Geometry: final body of the model. Coordinates: model frame, mm. Face numbers are marked on the shaded views. Give positions to 0.01 mm unless a question says otherwise; leave off trailing zeros. Order: outer loops, then holes, each group sorted by start corner. A loop starts at its lowest first (then second) coordinate and runs counter-clockwise, first axis right, second up. Notation, with made-up numbers: (25, -25.5) -> (29, -25.5) arc R26 ccw to (29, 13.5) -> close; hole circle Ø3 at (-3, 70.25). An arc over 180 degrees is marked (long way). One line per question, with ' | ' between items. Start each with the question number.
(1) First-contact query: pin 1 Ø3 at (y, z) = (24.15, 4.76) entering from +X; pin 2 Ø3.5 at (y, z) = (1.92, 4.76) entering from -X; pin 3 Ø1.5 at (y, z) = (24, 4) entering from -X. Flat tips, straight axial feed; report the tip coordinate or a pass-through.
(2) Mould query, pull axis X, two halves, no side actions, for the marked faces 1, 2 and 3. Classes: +X half, -X half, draft (parallel to the pull), parting line (faces both ways), or undercut.
(3) Section D-D (x = -211.5). Return loops of the section in (y, z) (1 decimal).
(4) Section B-B (y = 13.5). Return loops of the section in (x, z) (1 decimal), then the cut area to 3 significant figures.
(5) Section C-C (x = -220.5). Return loops of the section in (y, z) (1 decimal).
(6) Ray query, L1, parallel to Y at x = -223, z = 4.25; L2, parallel to Y at x = -245, z = 5.5; L3, parallel to X at y = 45, z = 3. Return the intervals inside material, ascending.
(7) Section A-A (z = 1.5). Return loops of the section in (x, y) (1 decimal).
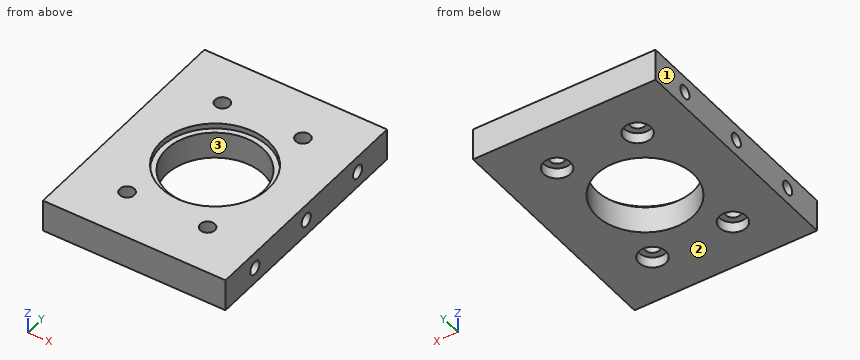
Autodesk Inventor part; units mm, degrees
ref_plane "Work Plane1" through (-222.5199, -10.7756, 0) normal (1, 0, 0) x (0, 0, -1)
ref_plane "YZ Plane" through (0, 0, 0) normal (1, 0, 0) x (0, 1, 0)
ref_plane "XZ Plane" through (0, 0, 0) normal (0, 1, 0) x (-1, 0, 0)
sketch "Sketch1" plane through (0, 0, 0) normal (0, 0, 1) x (1, 0, 0)
  circle A0 centre (0, 0) radius 38.1 construction
  circle A1 centre (0, 0) radius 41.275 construction
  line L0 (-7.3323, 0) -> (-3.6662, 6.35) construction
  line L1 (-3.6662, 6.35) -> (3.6662, 6.35) construction
  line L2 (3.6662, 6.35) -> (7.3323, 0) construction
  line L3 (7.3323, 0) -> (3.6662, -6.35) construction
  line L4 (3.6662, -6.35) -> (-3.6662, -6.35) construction
  line L5 (-3.6662, -6.35) -> (-7.3323, 0) construction
  circle A2 centre (0, 0) radius 14.2875 construction
  circle A3 centre (0, 0) radius 15.875 construction
  circle A4 centre (0, 0) radius 8.7313 construction
  circle A5 centre (0, 0) radius 22.225 construction
  line L6 (34.925, 38.1) -> (34.925, 95.25) construction
  line L7 (34.925, 95.25) -> (-34.925, 95.25) construction
  line L8 (-34.925, 95.25) -> (-34.925, 38.1) construction
  line L9 (34.925, 38.1) -> (-34.925, 38.1) construction
  line L10 (34.925, 38.1) -> (21.2491, -6.5137) construction
  line L11 (-34.925, 38.1) -> (-21.2491, -6.5137) construction
  circle A6 centre (-30.353, 38.1) radius 3.9624 construction
  line L12 (53.34, 95.25) -> (-53.34, 95.25) construction
  line L13 (-53.34, 95.25) -> (-53.34, 104.775) construction
  line L14 (-53.34, 104.775) -> (53.34, 104.775) construction
  line L15 (53.34, 104.775) -> (53.34, 95.25) construction
  circle A7 centre (-222.5199, 24.1494) radius 53.34 construction
  line L16 (-190.7699, 59.0744) -> (-254.2699, 59.0744)
  line L17 (-254.2699, 59.0744) -> (-254.2699, -10.7756)
  line L18 (-254.2699, -10.7756) -> (-190.7699, -10.7756)
  line L19 (-190.7699, -10.7756) -> (-190.7699, 59.0744)
  line L20 (-195.5324, 59.0744) -> (-195.5324, -10.7756)
  line L21 (-249.5074, 59.0744) -> (-249.5074, -10.7756)
  line L22 (-209.8199, 68.5994) -> (-235.2199, 68.5994) construction
  line L23 (-235.2199, 68.5994) -> (-235.2199, -20.3006) construction
  line L24 (-235.2199, -20.3006) -> (-209.8199, -20.3006) construction
  line L25 (-209.8199, -20.3006) -> (-209.8199, 68.5994) construction
  line L26 (34.925, 88.9) -> (-34.925, 88.9) construction
  circle A8 centre (30.353, 38.1) radius 3.9624 construction
  circle A9 centre (30.353, 76.2) radius 3.9624 construction
  circle A10 centre (-30.353, 76.2) radius 3.9624 construction
  circle A11 centre (0, 47.625) radius 3.9624 construction
  line L27 (34.925, 92.075) -> (-34.925, 92.075) construction
  circle A12 centre (0, 71.755) radius 14.2875 construction
  circle A13 centre (0, 71.755) radius 15.875 construction
  line L28 (7.3323, 71.755) -> (3.6662, 65.405) construction
  line L29 (3.6662, 65.405) -> (-3.6662, 65.405) construction
  line L30 (-3.6662, 65.405) -> (-7.3323, 71.755) construction
  line L31 (-7.3323, 71.755) -> (-3.6662, 78.105) construction
  line L32 (-3.6662, 78.105) -> (3.6662, 78.105) construction
  line L33 (3.6662, 78.105) -> (7.3323, 71.755) construction
  point P0 (22.225, 92.075)
  point P1 (0, 92.075)
  point P2 (-22.225, 92.075)
  point P3 (0, 47.625)
  dimension "d0" = 76.2
  dimension "d2" = 82.55
  dimension "d3" = 12.7
  dimension "d4" = 28.575
  dimension "d5" = 31.75
  dimension "d6" = 17.4625
  dimension "d7" = 44.45
  dimension "d8" = 69.85
  dimension "d9" = 34.925
  dimension "d10" = 38.1
  dimension "d11" = 57.15
  dimension "d13" = 7.9248
  dimension "d14" = 9.525
  dimension "d15" = 106.68
  dimension "d16" = 53.34
  dimension "d17" = 106.68
  dimension "d18" = 69.85
  dimension "d19" = 34.925
  dimension "d20" = 63.5
  dimension "d21" = 31.75
  dimension "d22" = 4.7625
  dimension "d23" = 4.7625
  dimension "d24" = 25.4
  dimension "d25" = 14.2875
  dimension "d26" = 88.9
  dimension "d27" = 14.2875
  dimension "d28" = 44.45
  dimension "d29" = 4.572
  dimension "d30" = 6.35
  dimension "d31" = 0
  dimension "d32" = 7.9248
  dimension "d33" = 4.572
  dimension "d34" = 7.9248
  dimension "d35" = 7.9248
  dimension "d36" = 4.572
  dimension "d37" = 4.572
  dimension "d38" = 38.1
  dimension "d39" = 38.1
  dimension "d40" = 7.9248
  dimension "d41" = 9.525
  dimension "d42" = 34.925
  dimension "d44" = 3.175
  dimension "d45" = 34.925
  dimension "d46" = 12.7
  dimension "d47" = 12.7
  dimension "d48" = 28.575
  dimension "d50" = 0
  dimension "d52" = 31.75
  dimension "d53" = 12.7
  dimension "d54" = 17.145
extrude "Plate1" add sketch "Sketch1" along normal blind 9.525 contours L20 L18 L21 L16
sketch "Sketch3" plane through (0, 0, 0) normal (0, 0, -1) x (-1, 0, 0)
  line L0 (249.5074, -10.7756) -> (195.5324, -10.7756)
  line L1 (249.5074, 59.0744) -> (249.5074, -10.7756)
  circle A0 centre (222.5199, 24.1494) radius 23.8125 construction
  line L2 (210.6137, 44.7716) -> (222.5199, 24.1494) construction
  line L3 (222.5199, 24.1494) -> (198.7074, 24.1494) construction
  point P0 (195.5324, 59.0744)
  point P1 (0, 0)
  point P2 (198.7074, 24.1494)
  point P3 (210.6137, 3.5271)
  point P4 (234.4262, 3.5271)
  point P5 (246.3324, 24.1494)
  point P6 (234.4262, 44.7716)
  dimension "d69" = 47.625
  dimension "d71" = 26.9875
  dimension "d72" = 53.975
  dimension "d73" = 34.925
  dimension "d74" = 69.85
  dimension "d75" = 60
  dimension "d78" = 360
hole "Hole2" at (-210.6137, 44.7716, 0) at (-210.6137, 3.5271, 0) at (-234.4262, 3.5271, 0) at (-234.4262, 44.7716, 0) direction (0, 0, 1) diameter 4.318 end through all counterbore diameter 7.9502 counterbore depth 3.175
sketch "Sketch4" plane through (0, 0, 9.525) normal (0, 0, 1) x (1, 0, 0)
  line L0 (-249.5074, -10.7756) -> (-249.5074, 59.0744)
  line L1 (-195.5324, -10.7756) -> (-249.5074, -10.7756)
  point P0 (0, 0)
  point P1 (-222.5199, 24.1494)
  dimension "d97" = 53.975
  dimension "d98" = 69.85
  dimension "d99" = 34.925
  dimension "d100" = 26.9875
hole "Hole4" at (-222.5199, 24.1494, 9.525) direction (0, 0, -1) diameter 28.575 end through all counterbore diameter 31.75 counterbore depth 1.5875
ref_plane "Work Plane1" through (-222.5199, -10.7756, 0) normal (1, 0, 0) x (0, 0, -1)
sketch "Sketch2" plane through (-195.5324, -10.7756, 0) normal (1, 0, 0) x (0, 0, -1)
  line L0 (0, 0) -> (-9.525, 0)
  line L1 (0, 69.85) -> (-9.525, 69.85)
  line L2 (-4.7625, 69.85) -> (-4.7625, 0) construction
  point P0 (0, 10.7756)
  point P1 (-4.7625, 57.15)
  point P2 (-4.7625, 34.925)
  point P3 (-4.7625, 12.7)
  dimension "d87" = 12.7
  dimension "d88" = 12.7
  dimension "d89" = 34.925
hole "Hole1" at (-195.5324, 46.3744, 4.7625) at (-195.5324, 24.1494, 4.7625) at (-195.5324, 1.9244, 4.7625) direction (-1, 0, 0) diameter 3.9624 depth 7.9375 tip angle 118
mirror "Mirror1" about plane through (-222.5199, -10.7756, 0) normal (1, 0, 0) of "Hole1"
equation "\"d19\" = 0.5 * d18"
equation "\"d21\" = 0.5 * d20"
equation "\"d22\" = d23"
equation "\"d25\" = d27"
equation "\"d28\" = 0.5 * d26"
equation "\"d32\" = d13"
equation "\"d33\" = d29"
equation "\"d34\" = d32"
equation "\"d35\" = d13"
equation "\"d36\" = d29"
equation "\"d37\" = d29"
equation "\"d39\" = d38"
equation "\"d40\" = d13"
equation "\"d44\" = 0.5 * d30"
equation "\"d71\" = 0.5 * d72"
equation "\"d73\" = 0.5 * d74"
equation "\"d106\" = Thickness"
equation "\"BendRadius\" = Thickness"
equation "\"BendReliefWidth\" = Thickness"
equation "\"BendReliefDepth\" = 0.5 * Thickness"
equation "\"CornerReliefSize\" = 4 * Thickness"
equation "\"MinimumRemnant\" = 2 * Thickness"
equation "\"TransitionRadius\" = BendRadius"
equation "\"JacobiRadiusSize\" = Thickness"
equation "\"GapSize\" = Thickness"
equation "\"d55\" = BendRadius"
properties part number "Swerve Wheel + Carriage Outline V1"
Response:
1) pin 1: stops at x = -203.76 | pin 2: stops at x = -241.43 | pin 3: stops at x = -241.3
2) face 1: -X half | face 2: draft | face 3: undercut
3) outline: (-10.8, 0) -> (-0.3, 0) -> (-0.3, 3.2) -> (1.6, 3.2) -> (1.6, 9.5) -> (-10.8, 9.5) -> close; (5.5, 3.2) -> (7.4, 3.2) -> (7.4, 0) -> (15.1, 0) -> (15.1, 7.9) -> (12.7, 7.9) -> (12.7, 9.5) -> (5.5, 9.5) -> close; (33.2, 0) -> (40.9, 0) -> (40.9, 3.2) -> (42.8, 3.2) -> (42.8, 9.5) -> (35.6, 9.5) -> (35.6, 7.9) -> (33.2, 7.9) -> close; (46.7, 3.2) -> (48.6, 3.2) -> (48.6, 0) -> (59.1, 0) -> (59.1, 9.5) -> (46.7, 9.5) -> close
4) outline: (-249.5, 0) -> (-232, 0) -> (-232, 7.9) -> (-234.3, 7.9) -> (-234.3, 9.5) -> (-249.5, 9.5) -> close; (-213, 0) -> (-195.5, 0) -> (-195.5, 9.5) -> (-210.7, 9.5) -> (-210.7, 7.9) -> (-213, 7.9) -> close | area: 326 mm^2
5) outline: (-10.8, 0) -> (10, 0) -> (10, 7.9) -> (8.4, 7.9) -> (8.4, 9.5) -> (-10.8, 9.5) -> close; (38.3, 0) -> (59.1, 0) -> (59.1, 9.5) -> (39.9, 9.5) -> (39.9, 7.9) -> (38.3, 7.9) -> close
6) L1: y = -10.78 to 9.87, 38.43 to 59.07 | L2: y = -10.78 to 0.09, 3.76 to 22.31, 25.99 to 44.54, 48.21 to 59.07 | L3: x = -249.51 to -238.39, -230.46 to -214.58, -206.65 to -195.53
7) outline: (-249.5, -10.8) -> (-195.5, -10.8) -> (-195.5, 59.1) -> (-249.5, 59.1) -> close; hole circle Ø8 at (-234.4, 3.5); hole circle Ø8 at (-234.4, 44.8); hole circle Ø28.6 at (-222.5, 24.1); hole circle Ø8 at (-210.6, 3.5); hole circle Ø8 at (-210.6, 44.8)
